Could you check a few things on this model? Use its own coordinates, in mm. A direction names the side the tool comes from. Give positions to 0.01 mm unless a question says otherwise; leave off trailing zeros. Loops run counter-clockwise (first coordinate to the right, second up) from the corner with the lowest first, then second, coordinate; pieces in that order, holes last. Notation, with made-up numbers: M 87.25,42.25 L 128.25,42.25 A14 ccw 128.25,57.25 Z; hole C -18,-7.75 d4. An arc over 180 degrees is marked long. Use CSV: the item, a comma, the result in double quotes.
Autodesk Inventor part; units mm, degrees
ref_plane "YZ Plane" through (0, 0, 0) normal (1, 0, 0) x (0, 1, 0)
ref_plane "XZ Plane" through (0, 0, 0) normal (0, 1, 0) x (-1, 0, 0)
ref_plane "XY Plane" through (0, 0, 0) normal (0, 0, 1) x (1, 0, 0)
sketch "Sketch1" plane through (0, 0, 0) normal (0, 0, 1) x (1, 0, 0)
  line L0 (-40.6, 40.6) -> (51.4, 40.6)
  line L1 (51.4, 40.6) -> (51.4, -40.6)
  line L2 (51.4, -40.6) -> (-40.6, -40.6)
  line L3 (-40.6, -40.6) -> (-40.6, 40.6)
  line L4 (-42.6, 42.6) -> (53.4, 42.6)
  line L5 (53.4, 42.6) -> (53.4, -42.6)
  line L6 (53.4, -42.6) -> (-42.6, -42.6)
  line L7 (-42.6, -42.6) -> (-42.6, 42.6)
  point P0 (0, 0)
  dimension "d0" = 92
  dimension "d1" = 81.2
  dimension "d2" = 40.6
  dimension "d3" = 40.6
  dimension "d4" = 2
  dimension "d5" = 2
  dimension "d6" = 2
  dimension "d7" = 2
extrude "Extrusion1" add sketch "Sketch1" along normal blind 40
properties part number "expected_size"
1. I want a section at C-C, the plane x = -17. List the corners of the cut face in (y, z) for me, then the cut area to 3 significant figures.
Outcome:
outline,"M -42.6,0 L -40.6,0 L -40.6,40 L -42.6,40 Z; M 40.6,0 L 42.6,0 L 42.6,40 L 40.6,40 Z"
area,"160 mm2"
2. If we mould it in two halves opening along X, with no side actions, what happens to faces 3 (the face through (-42.6, -1, 20)), 4 (the face through (53.4, 1, 20)), 5 (the face through (51.4, 1, 20))? For each: +X half, -X half, draft (parallel to the pull), parting line (faces both ways), or undercut.
Outcome:
face 3,"-X half"
face 4,"+X half"
face 5,"undercut"
3. I want a section at B-B, the plane z = 25. List the corners of the cut face in (x, y) for me, then the cut area to 3 significant figures.
Outcome:
outline,"M -42.6,-42.6 L 53.4,-42.6 L 53.4,42.6 L -42.6,42.6 Z; hole M -40.6,-40.6 L 51.4,-40.6 L 51.4,40.6 L -40.6,40.6 Z"
area,"709 mm2"
4. Please list where these lines run through material, in increasing order: line 1 (Y direction, x = 42.5, z = 33); line 2 (X direction, y = -24, z = 23).
Outcome:
line 1,"-42.6 to -40.6, 40.6 to 42.6"
line 2,"-42.6 to -40.6, 51.4 to 53.4"
5. I want a section at A-A, the plane y = 37.5. List the corners of the cut face in (x, z) for me.
Outcome:
outline,"M -42.6,0 L -40.6,0 L -40.6,40 L -42.6,40 Z; M 51.4,0 L 53.4,0 L 53.4,40 L 51.4,40 Z"
6. Which directions (+Z, -Z, +X, -X, +Y, -Y) give clear straight access to the entire face, cutting with the end or side of a thin tool? Please do faces 1 (the face through (-40.6, -1, 20)), 2 (the face through (6, -42.6, 20)).
Outcome:
face 1,"+Z, -Z"
face 2,"+Z, -Z, +X, -X, -Y"
